Could you check a few things on this model? Use its own coordinates, in mm. A direction names the side the tool comes from. Round coordinates to 2 decimals unless told otherwise and drop trailing zeros. Loops run counter-clockwise (first coordinate to the right, second up) from the corner with the lowest first, then second, coordinate; pieces in that order, holes last.
Autodesk Inventor part; units mm, degrees
ref_plane "Start plane" through (0, 0, 0) normal (0, 0, 1) x (1, 0, 0)
ref_plane "End plane" through (0, 0, 177.8) normal (0, 0, 1) x (1, 0, 0)
ref_plane "YZ Plane" through (0, 0, 0) normal (1, 0, 0) x (0, 1, 0)
ref_plane "Start plane" through (0, 0, 0) normal (0, 0, 1) x (1, 0, 0)
ref_plane "End plane" through (0, 0, 177.8) normal (0, 0, 1) x (1, 0, 0)
sketch "Sketch" plane through (0, 0, 0) normal (0, 0, 1) x (1, 0, 0)
  line L0 (-12.5, -8.75) -> (-12.5, 8.75)
  line L1 (-8.75, 12.5) -> (8.75, 12.5)
  line L2 (12.5, 8.75) -> (12.5, -8.75)
  line L3 (8.75, -12.5) -> (-8.75, -12.5)
  arc A0 (-12.5, -8.75) -> (-8.75, -12.5) centre (-8.75, -8.75) ccw
  arc A1 (-8.75, 12.5) -> (-12.5, 8.75) centre (-8.75, 8.75) ccw
  arc A2 (12.5, 8.75) -> (8.75, 12.5) centre (8.75, 8.75) ccw
  arc A3 (8.75, -12.5) -> (12.5, -8.75) centre (8.75, -8.75) ccw
  arc A4 (-8.75, 10) -> (-10, 8.75) centre (-8.75, 8.75) ccw
  line L4 (-8.75, 10) -> (8.75, 10)
  arc A5 (10, 8.75) -> (8.75, 10) centre (8.75, 8.75) ccw
  line L5 (10, 8.75) -> (10, -8.75)
  arc A6 (8.75, -10) -> (10, -8.75) centre (8.75, -8.75) ccw
  line L6 (8.75, -10) -> (-8.75, -10)
  arc A7 (-10, -8.75) -> (-8.75, -10) centre (-8.75, -8.75) ccw
  line L7 (-10, -8.75) -> (-10, 8.75)
  line L8 (0, 18.5873) -> (0, -18.5873) construction
  line L9 (-18.5873, 0) -> (18.5873, 0) construction
  dimension "d7" = 3.75
  dimension "d10" = 25
  dimension "d11" = 25
  dimension "d12" = 2.5
  dimension "d15" = 12.5
  dimension "d16" = 12.5
extrude "Body" add sketch "Sketch" along normal up to surface (177.8 mm away) from surface at 0
sketch "Sketch3" plane through (0, 0, 0) normal (0, 0, 1) x (1, 0, 0)
  line L0 (0, 0) -> (10, 0)
ref_plane "Work Plane3" through (0, 0, 0) normal (0, -1, 0) x (1, 0, 0)
sketch "Sketch4" plane through (0, 0, 0) normal (0, -1, 0) x (1, 0, 0)
  line L0 (-2, 0) -> (12, 0)
  line L1 (-2, 177.8) -> (12, 177.8)
  dimension "d18" = 177.8
equation "\"d7\" = G_IR"
equation "\"d10\" = G_H"
equation "\"d11\" = G_W"
equation "\"d12\" = G_T"
equation "\"d15\" = 0.5 * d10"
equation "\"d16\" = 0.5 * d11"
equation "\"d3\" = G_L"
equation "\"G_W\" = 25"
equation "\"G_H\" = 25"
equation "\"G_T\" = 2.5"
equation "\"G_IR\" = 3.75"
equation "\"G_L\" = d18"
equation "\"G_OFFSET_START\" = 0"
equation "\"G_OFFSET_END\" = 0"
equation "\"d14\" = G_OFFSET_END + B_L"
equation "\"B_L\" = 177.8"
properties part number "ISO 25x25x2.5 00000001"
Item 1: Will this pin go through, and if not, where does the flat tip stop? pin 1 (1 mm diameter, centred on y = -9.5, z = 157.5, fed in from -X).
Results list:
pin 1: stops at x = -12.49
Item 2: If we section it at C-C, the plane z = 16.5: Please give me the cut outline in (x, y), then the cut area to 3 significant figures.
Results list:
outline: (-12.5, -8.75) arc R3.75 ccw to (-8.75, -12.5) - (8.75, -12.5) arc R3.75 ccw to (12.5, -8.75) - (12.5, 8.75) arc R3.75 ccw to (8.75, 12.5) - (-8.75, 12.5) arc R3.75 ccw to (-12.5, 8.75) - close; hole (-10, -8.75) arc R1.25 ccw to (-8.75, -10) - (8.75, -10) arc R1.25 ccw to (10, -8.75) - (10, 8.75) arc R1.25 ccw to (8.75, 10) - (-8.75, 10) arc R1.25 ccw to (-10, 8.75) - close
area: 214 mm2
Item 3: If we section it at A-A, the plane x = 6: Please give me the cut outline in (y, z), then the cut area to 3 significant figures.
Results list:
outline: (-12.5, 0) - (-10, 0) - (-10, 177.8) - (-12.5, 177.8) - close; (10, 0) - (12.5, 0) - (12.5, 177.8) - (10, 177.8) - close
area: 889 mm2
Item 4: We'd pull the mould along Y, two halves only. Please class faces 1 (the flat face through (10, 0, 88)), 2 (the flat face through (-11, 0, 0)), 3 (the cylindrical face through (11.372, 11.431, 87.655)), 4 (the flat face through (0, -10, 88)): released by +Y, released by -Y, zero draft, split by the parting line, or undercut.
Results list:
face 1: undercut
face 2: zero draft
face 3: released by +Y
face 4: undercut
Item 5: For faces 5 (the flat face through (0, -12.5, 88)), 6 (the flat face through (-10, 0, 88)), which set-ups out of +Z, -Z, +X, -X, +Y, -Y let a thin tool reach every point of the face, with its end or its side?
Results list:
face 5: +Z, -Z, +X, -X, -Y
face 6: +Z, -Z
Item 6: If I drill on line 1 along Y through (x, z) = (1.5, 149.5); line 2 along Y through (x, z) = (11, 94.5), over which ranges is the centre line in solid material (lowest first)?
Results list:
line 1: y = -12.5 to -10, 10 to 12.5
line 2: y = -11.75 to 11.75
